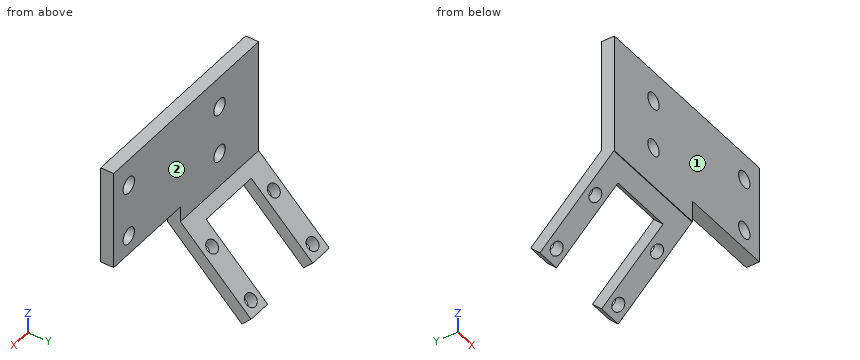
```python
from build123d import *

# Parameters (mm, degrees)
SKETCH2_W           = 48.15
SKETCH2_H           = 26.520901759
SKETCH2_R           = 1.89
BOSS_EXTRUDE1_DEPTH = 3
SKETCH6_R           = 1.5
BOSS_EXTRUDE2_DEPTH = 3
SKETCH7_W           = 26
SKETCH7_H           = 2.377108006
BOSS_EXTRUDE3_DEPTH = 2
SKETCH8_W           = 22.15
SKETCH8_H           = 3.609216989
CUT_EXTRUDE1_DEPTH  = 3


with BuildPart() as part:
    # Sketch2 → Boss-Extrude1 (new body)
    with BuildSketch(Plane(origin=(0, 0, 0), x_dir=(1, 0, 0), z_dir=(0, 1, 0))):
        with Locations((-4, -2.085450879)):
            Rectangle(SKETCH2_W, SKETCH2_H)
        with Locations((-15.075, -8.175)):
            Circle(SKETCH2_R, mode=Mode.SUBTRACT)
        with Locations((-15.075, 3.175)):
            Circle(SKETCH2_R, mode=Mode.SUBTRACT)
        with Locations((15.075, 3.175)):
            Circle(SKETCH2_R, mode=Mode.SUBTRACT)
        with Locations((15.075, -9.175)):
            Circle(SKETCH2_R, mode=Mode.SUBTRACT)
    extrude(amount=BOSS_EXTRUDE1_DEPTH)

    # Sketch6 → Boss-Extrude2 (add)
    with BuildSketch(Plane(origin=(0, -4.0875, -4.0875), x_dir=(-1, 0, 0), z_dir=(0, -0.707106781, -0.707106781))):
        Polygon((2.075, 8.962578452), (28.075, 8.962578452), (28.075, 33), (22.575, 33), (22.575, 13), (7.575, 13), (7.575, 33), (2.075, 33), align=None)
        with Locations((4.825, 17.65)):
            Circle(SKETCH6_R, mode=Mode.SUBTRACT)
        with Locations((25.325, 17.65)):
            Circle(SKETCH6_R, mode=Mode.SUBTRACT)
        with Locations((4.825, 30.25)):
            Circle(SKETCH6_R, mode=Mode.SUBTRACT)
        with Locations((25.325, 30.25)):
            Circle(SKETCH6_R, mode=Mode.SUBTRACT)
    extrude(amount=BOSS_EXTRUDE2_DEPTH)

    # Sketch7 → Boss-Extrude3 (add)
    with BuildSketch(Plane.XZ):
        with Locations((-15.075, -11.357766341)):
            Rectangle(SKETCH7_W, SKETCH7_H)
    extrude(amount=-BOSS_EXTRUDE3_DEPTH)

    # Sketch8 → Cut-Extrude1 (cut)
    with BuildSketch(Plane(origin=(0, 3, 0), x_dir=(1, 0, 0), z_dir=(0, 1, 0))):
        with Locations((9, 9.370391506)):
            Rectangle(SKETCH8_W, SKETCH8_H)
    extrude(amount=-CUT_EXTRUDE1_DEPTH, mode=Mode.SUBTRACT)


solid = part.part
```
Here's how the part is built. I have some questions about the finished solid (model axes, mm). Face numbers are marked on the shaded views. A direction names the side the tool comes from. Round coordinates to 2 decimals unless told otherwise and drop trailing zeros. Order: outer loops, then holes, each group sorted by start corner. A loop starts at its lowest first (then second) coordinate and runs counter-clockwise, first axis right, second up. Notation, with made-up numbers: M -2,-29.75 L 57,-29.75 A23 ccw 57,-16.75 Z; hole C -35,-2 d10. An arc over 180 degrees is marked long. Use CSV: the item, a comma, the result in double quotes.
1) I want a section at A-A (x = 14). List the corners of the cut face in (y, z) for me.
Taken from the geometry:
outline,"M 0,-7.57 L 3,-7.57 L 3,-4.73 L 0,-4.73 Z; M 0,-1.62 L 3,-1.62 L 3,7.62 L 0,7.62 Z; M 0,10.73 L 3,10.73 L 3,15.35 L 0,15.35 Z"
2) I'm going to push flat-ended pins straight in: P1, Ø8, axis at y = 9.5, z = -22, coming from the +X side (3 decimals); P2, Ø12, axis at x = -17.5, z = -19.5, coming from the -Y side; P3, Ø6, axis at x = -21, y = 11.5, coming from the -Z side. Where does each tip first touch, or does it pass through?
Taken from the geometry:
P1,"x = -2.075"
P2,"y = 1.08"
P3,"z = -26.47"
3) I want a section at C-C (x = -10). List the corners of the cut face in (y, z) for me (3 decimals).
Taken from the geometry:
outline,"M 0,-12.546 L 0.129,-12.546 L 2.984,-15.401 L 5.105,-13.28 L 3,-11.175 L 3,15.346 L 0,15.346 Z"
4) I want a section at D-D (z = -10.5). List the corners of the cut face in (x, y) for me (3 decimals).
Taken from the geometry:
outline,"M -28.075,0 L -2.075,0 L -2.075,3 L -28.075,3 Z"
5) I need wall thicknesses on line 1 along Z through (x, y) = (-15, 2); line 2 along Y through (x, z) = (-17.5, 9.5); line 3 along Z through (x, y) = (-10, 4) (3 decimals). Which ranges of each line are inside material? Lowest first, please. Write a range as [from, to].
Taken from the geometry:
line 1,"[-14.42, -5.06], [-1.29, 6.29], [10.06, 15.35]"
line 2,"[0, 3]"
line 3,"[-14.385, -12.175]"
6) On a 3-axis mill with a long thin cutter (end or side, diameter ignored), from which of +Z, -Z, +X, -X, +Y, -Y can I reach the whole of each face in a straight line? I mean the marked faces 1 and 2. Say none if no direction works.
Taken from the geometry:
face 1,"+Z, -Z, +X, -X, -Y"
face 2,"+Z, +X, -X, +Y"
7) I want a section at B-B (y = 2.25). List the corners of the cut face in (x, z) for me (3 decimals), then the cut area to 3 significant figures.
Taken from the geometry:
outline,"M -28.075,-14.668 L -2.075,-14.668 L -2.075,-7.566 L 20.075,-7.566 L 20.075,15.346 L -28.075,15.346 Z; hole C -15.075,-3.175 d3.78; hole C -15.075,8.175 d3.78; hole C 15.075,-3.175 d3.78; hole C 15.075,9.175 d3.78"
area,"1,240 mm^2"
